Geometry check sheet. Reference: the model listing, model coordinates, mm. A direction names the side the tool comes from. Round coordinates to 2 decimals unless told otherwise and drop trailing zeros. Loops run counter-clockwise (first coordinate to the right, second up) from the corner with the lowest first, then second, coordinate; pieces in that order, holes last. Notation, with made-up numbers: M 34,57 L 74,57 A14 ccw 74,75 Z; hole C -26.5,-14 d4. An arc over 180 degrees is marked long. Write item = value, one per line.
from build123d import *

# Parameters (mm, degrees)
SKETCH_1_W          = 60
SKETCH_1_H          = 20
SKETCH_1_R          = 2.55
EXTRUDE_1_DEPTH     = 5
SKETCH_3_W          = 22
SKETCH_3_H          = 20
EXTRUDE_2_DEPTH     = 16
SKETCH_4_R          = 15
EXTRUDE_3_DEPTH     = 20
SKETCH_5_R          = 4.25
CUT_EXTRUDE_1_DEPTH = 58.374334501
SKETCH_6_R          = 11.1
CUT_EXTRUDE_2_DEPTH = 8


with BuildPart() as part:
    # 草图1 → 凸台-拉伸1 (new body)
    with BuildSketch(Plane(origin=(0, 0, 0), x_dir=(1, 0, 0), z_dir=(0, 1, 0))):
        with Locations((9.947643979, -4.502617801)):
            Rectangle(SKETCH_1_W, SKETCH_1_H)
        with Locations(Location((-12.052356021, -4.502617801, 0), (0, 0, 270))):
            Circle(SKETCH_1_R, mode=Mode.SUBTRACT)
        with Locations(Location((31.947643979, -4.502617801, 0), (0, 0, 270))):
            Circle(SKETCH_1_R, mode=Mode.SUBTRACT)
    extrude(amount=EXTRUDE_1_DEPTH)

    # 草图3 → 凸台-拉伸2 (add)
    with BuildSketch(Plane(origin=(0, 5, 0), x_dir=(1, 0, 0), z_dir=(0, 1, 0))):
        with Locations((9.947643979, -4.502617801)):
            Rectangle(SKETCH_3_W, SKETCH_3_H)
    extrude(amount=EXTRUDE_2_DEPTH)

    # 草图4 → 凸台-拉伸3 (add)
    with BuildSketch(Plane(origin=(0, 0, -5.497382199), x_dir=(-1, 0, 0), z_dir=(0, 0, -1))):
        with Locations((-9.947643979, 21)):
            Circle(SKETCH_4_R)
    extrude(amount=-EXTRUDE_3_DEPTH)

    # 草图5 → 切除-拉伸1 (cut, through all)
    with BuildSketch(Plane.XY.offset(14.502617801)):
        with Locations((9.947643979, 21)):
            Circle(SKETCH_5_R)
    extrude(amount=-CUT_EXTRUDE_1_DEPTH, mode=Mode.SUBTRACT)

    # 草图6 → 切除-拉伸2 (cut)
    with BuildSketch(Plane.XY.offset(14.502617801)):
        with Locations((9.947643979, 21)):
            Circle(SKETCH_6_R)
    extrude(amount=-CUT_EXTRUDE_2_DEPTH, mode=Mode.SUBTRACT)


solid = part.part
(1) Tool access check on faces 4 (the flat face through (20.948, 8, 5)), 5 (the cylindrical face through (9.461, 35.992, 4.363)), 6 (the flat face through (15, 21, 6.503)), 7 (the flat face through (-1.052, 8, 5)). Record the directions out of +Z, -Z, +X, -X, +Y, -Y that give a thin tool (end or side, any length) a straight path to the whole face; none if there is none.
Result set:
face_4 = +Z, -Z, +X
face_5 = +Z, -Z
face_6 = +Z
face_7 = +Z, -Z, -X
(2) Sectioned sample at B-B on y = 21. Record the cut outline in (x, z).
Result set:
outline = M -5.05,-5.5 L 5.7,-5.5 L 5.7,6.5 L -1.15,6.5 L -1.15,14.5 L -5.05,14.5 Z; M 14.2,-5.5 L 24.95,-5.5 L 24.95,14.5 L 21.05,14.5 L 21.05,6.5 L 14.2,6.5 Z
(3) Sectioned sample at C-C on z = -2.5. Record the cut outline in (x, y), then the cut area to 3 significant figures.
Result set:
outline = M -20.05,0 L 39.95,0 L 39.95,5 L 20.95,5 L 20.95,10.8 A15 ccw long -1.05,10.8 L -1.05,5 L -20.05,5 Z; hole C 9.95,21 d8.5
area = 1,000 mm2
(4) Sectioned sample at D-D on y = 14. Record the cut outline in (x, z), then the cut area to 3 significant figures.
Result set:
outline = M -3.32,-5.5 L 23.21,-5.5 L 23.21,14.5 L 18.56,14.5 L 18.56,6.5 L 1.33,6.5 L 1.33,14.5 L -3.32,14.5 Z
area = 393 mm2
(5) Depth check by flat-ended pin: pin 1 Ø8 at (y, z) = (19, 9) entering from -X; pin 2 Ø1.7 at (y, z) = (8, 5) entering from +X; pin 3 Ø8 at (x, z) = (31.95, 4.5) entering from +Y; pin 4 Ø12 at (x, y) = (-13.5, 17) entering from +Z. Enter the tip coordinate at first touch or a pass-through.
Result set:
pin_1 = -5.05
pin_2 = 20.95
pin_3 = 5
pin_4 = through
(6) Material ranges on line 1 along Y through (x, z) = (9.5, 8.75); line 2 along Y through (x, z) = (8, 7.75); line 3 along Y through (x, z) = (-15, 3.75), recorded low to high. Write a range as from..to.
Result set:
line_1 = 0..9.91, 32.09..35.99
line_2 = 0..10.07, 31.93..35.87
line_3 = 0..5
(7) Sectioned sample at A-A on z = 10.75. Record the cut outline in (x, y).
Result set:
outline = M -20.05,0 L 39.95,0 L 39.95,5 L 20.95,5 L 20.95,10.8 A15 ccw long -1.05,10.8 L -1.05,5 L -20.05,5 Z; hole C 9.95,21 d22.2
(8) Release check for a two-part mould opening along Z. For faces 1 (the cylindrical face through (29.46, 2.46, 3.95)), 2 (the flat face through (28, 5, 4)), 3 (the flat face through (10, 9, 14.503)) record: released by +Z, released by -Z, zero draft, split by the parting line, or undercut.
Result set:
face_1 = undercut
face_2 = zero draft
face_3 = released by +Z
